Could you check a few things on this drawing? It's one solid part, dimensions in mm from its lowest x, y, z. Round coordinates to 2 decimals unless told otherwise and drop trailing zeros. Loops run counter-clockwise (first coordinate to the right, second up) from the corner with the lowest first, then second, coordinate; pieces in that order, holes last.
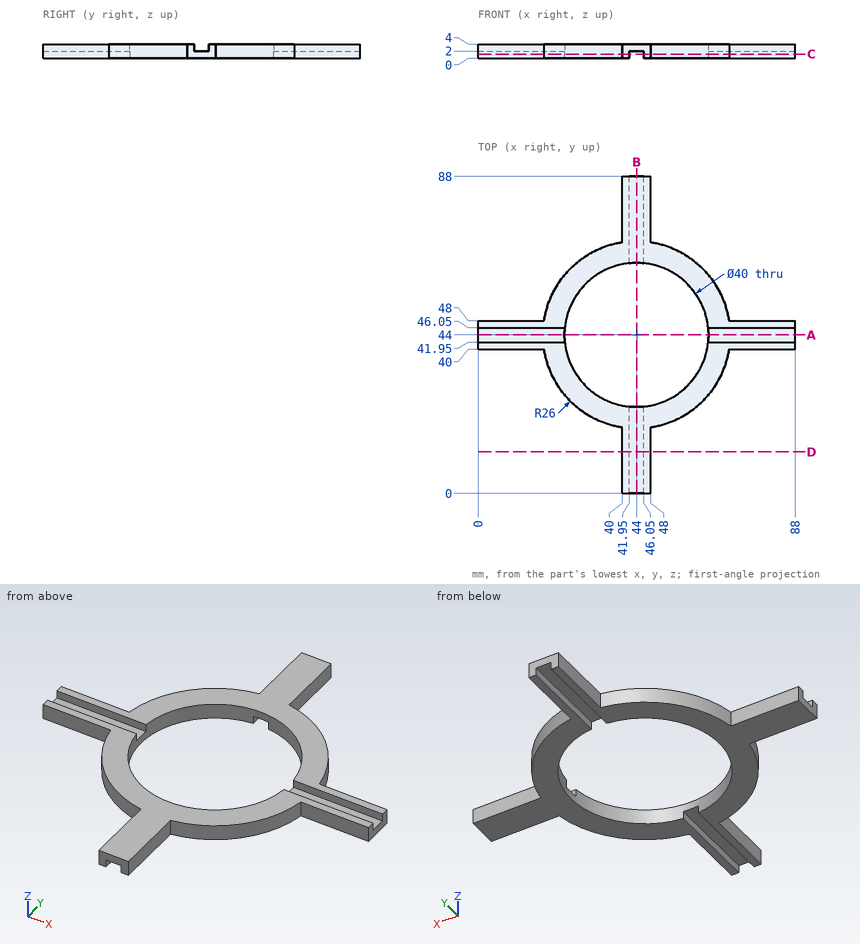
(1) If I drill on line 1 (X direction, y = 6, z = 0.55); line 2 (Y direction, x = 44, z = 2.85), over which ranges is the centre line in solid material (lowest first)?
(2) Suppose I cut it at C-C (z = 1.2). Write out the boundary of the cut face in (x, y).
(3) Suppose I cut it at D-D (y = 11.5). Write out the boundary of the cut face in (x, z), then the cut area to 3 significant figures.
(4) Suppose I cut it at A-A (y = 44). Write out the boundary of the cut face in (x, z), then the cut area to 3 significant figures.
(5) Suppose I cut it at B-B (x = 44). Write out the boundary of the cut face in (y, z).
(6) For pin 1 (1 mm diameter, centred on y = 15, z = 1, fed in from +X); pin 2 (2 mm diameter, centred on x = 74, z = 2.5, fed in from +Y); pin 3 (1.2 mm diameter, centred on x = 7, y = 43, fed in from +Z), each with a flat end and sliding along its axis, tell me the tip position at first contact or that it passes through.
Check result:
1. line 1: x = 40 to 41.95, 46.05 to 48
1. line 2: y = 0 to 24, 64 to 88
2. outline: (0, 40) - (18.31, 40) arc R26 ccw to (40, 18.31) - (40, 0) - (41.95, 0) - (41.95, 24.11) arc R20 cw to (41.95, 63.89) - (41.95, 88) - (40, 88) - (40, 69.69) arc R26 ccw to (18.31, 48) - (0, 48) - close; (46.05, 0) - (48, 0) - (48, 18.31) arc R26 ccw to (69.69, 40) - (88, 40) - (88, 48) - (69.69, 48) arc R26 ccw to (48, 69.69) - (48, 88) - (46.05, 88) - (46.05, 63.89) arc R20 cw to (46.05, 24.11) - close
3. outline: (40, 0) - (41.95, 0) - (41.95, 2) - (46.05, 2) - (46.05, 0) - (48, 0) - (48, 4) - (40, 4) - close
3. area: 23.8 mm2
4. outline: (0, 0) - (24, 0) - (24, 2) - (0, 2) - close; (64, 0) - (88, 0) - (88, 2) - (64, 2) - close
4. area: 96.0 mm2
5. outline: (0, 2) - (24, 2) - (24, 4) - (0, 4) - close; (64, 2) - (88, 2) - (88, 4) - (64, 4) - close
6. pin 1: stops at x = 48
6. pin 2: stops at y = 48
6. pin 3: stops at z = 2
